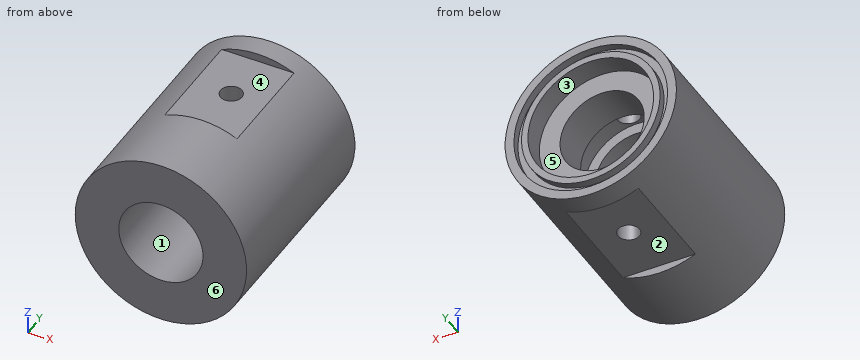
Autodesk Inventor part; units mm, degrees
ref_plane "YZ Plane" through (0, 0, 0) normal (1, 0, 0) x (0, 1, 0)
ref_plane "XZ Plane" through (0, 0, 0) normal (0, 1, 0) x (-1, 0, 0)
ref_plane "XY Plane" through (0, 0, 0) normal (0, 0, 1) x (1, 0, 0)
sketch "Sketch1" plane through (0, 0, 0) normal (0, 1, 0) x (-1, 0, 0)
  circle A0 centre (0, 0) radius 16
  dimension "d0" = 32
extrude "Extrusion1" add sketch "Sketch1" along normal blind 38
thread "Thread1"
sketch "Sketch2" plane through (0, 0, 0) normal (0, -1, 0) x (1, 0, 0)
  circle A0 centre (0, 0) radius 7.875
  dimension "d5" = 15.75
extrude "Extrusion2" cut sketch "Sketch2" against normal through all
sketch "Sketch3" plane through (0, 38, 0) normal (0, 1, 0) x (1, 0, 0)
  circle A0 centre (0, 0) radius 11.75
  dimension "d8" = 23.5
extrude "Extrusion3" cut sketch "Sketch3" against normal blind 4
sketch "Sketch4" plane through (0, 0, 0) normal (1, 0, 0) x (0, 1, 0)
  line L0 (0, 16) -> (38, 16)
  line L1 (34, 16) -> (14, 16)
  line L2 (14, 16) -> (14, 14.5)
  line L3 (14, 14.5) -> (34, 14.5)
  line L4 (34, 14.5) -> (34, 16)
  line L5 (0, -16) -> (38, -16)
  line L6 (34, -16) -> (14, -16)
  line L7 (14, -16) -> (14, -14.5)
  line L8 (14, -14.5) -> (34, -14.5)
  line L9 (34, -14.5) -> (34, -16)
  line L10 (38, -16) -> (38, 16)
  point P0 (0, 0)
  point P1 (14, 16)
  point P2 (14, -16)
  dimension "d11" = 20
  dimension "d12" = 1.5
  dimension "d13" = 1.5
  dimension "d33" = 4
extrude "Extrusion4" cut sketch "Sketch4" along normal through all both and the other way through all
sketch "Sketch5" plane through (0, 0, 0) normal (0, 0, 1) x (1, 0, 0)
  line L0 (7.875, 0) -> (7.875, 34)
  line L1 (7.875, 26.75) -> (9.875, 26.75)
  line L2 (9.875, 26.75) -> (9.875, 21.75)
  line L3 (9.875, 21.75) -> (7.875, 21.75)
  line L4 (7.875, 21.75) -> (7.875, 26.75)
  line L5 (0, -5.7834) -> (0, 45.928)
  line L6 (-11.75, 38) -> (11.75, 38)
  point P0 (0, 0)
  point P1 (7.875, 21.75)
  dimension "d17" = 11.25
  dimension "d18" = 16.25
  dimension "d19" = 2
revolve "Revolution1" cut sketch "Sketch5" angle 360 about axis through (0, -5.7834, 0) along (0, 1, 0)
sketch "Sketch6" plane through (6.7639, 34, -14.5) normal (0, 0, -1) x (-1, 0, 0)
  line L0 (-3.1111, -7.25) -> (16.6389, -7.25)
  line L1 (-3.1111, -12.25) -> (16.6389, -12.25)
  point P0 (6.7639, -34)
  point P1 (6.5383, -9.75)
  dimension "d20" = 5
  dimension "d21" = 2.5
hole "Hole1" at (0.2255, 24.25, -14.5) direction (0, 0, 1) diameter 4 end through all
sketch "Sketch7" plane through (0, 38, 0) normal (0, 1, 0) x (1, 0, 0)
  circle A0 centre (0, 0) radius 12.95
  circle A1 centre (0, 0) radius 14.35
  circle A2 centre (0, 0) radius 11.75
  dimension "d29" = 1.2
  dimension "d30" = 1.4
extrude "Extrusion5" cut sketch "Sketch7" against normal blind 1.4 contours A1
properties part number "Passthrough Base Insert" material "Aluminum 6061"
Can you work these out from the model? Positions are in its coordinate system, mm. Face numbers are marked on the shaded views. A direction names the side the tool comes from. Coordinates: 2 decimals unless noted, no trailing zeros. Loops run counter-clockwise (first coordinate to the right, second up) from the corner with the lowest first, then second, coordinate; pieces in that order, holes last. Notation, with made-up numbers: (85.5, 67) - (93.5, 67) arc R17 ccw to (93.5, 97) - close; hole circle Ø6 at (64, 11.25). An arc over 180 degrees is marked (long way). Answer as CSV lines item,"result". Start each with the question number.
1) Suppose I cut it at D-D (x = -1). Count the separate pieces of the cut face and the enclosed holes in it, plus the area to 3 significant figures.
2) Thinking about a two-plate mould opening in Z: for the marked faces 1, 2, 3 and 4, which applies, pulls with the +Z half, pulls with the -Z half, needs draft (parallel to the pull), parting line crosses it, or undercut?
3) Suppose I cut it at A-A (z = 0). Please give me the cut outline in (x, y) (3 decimals).
4) I need wall thicknesses on line 1 (Z direction, x = -0.5, y = 36.5); line 2 (Z direction, x = 0, y = 28) (3 decimals); line 3 (Y direction, x = -5.5, z = 6.5). Which ranges of each line are inside material? Lowest first, please. Write a range as from..to.
5) For pin 1 (0.5 mm diameter, centred on x = -2, z = 15, fed in from -Y); pin 2 (3 mm diameter, centred on x = 8.5, y = 15, fed in from -Z); pin 3 (5 mm diameter, centred on x = -13, y = 17.5, fed in from +Z); pin 4 (1.5 mm diameter, centred on y = 5, z = -4, fed in from -X), each with a flat end and sliding along its axis, tell me the tip position at first contact or that it passes through.
6) Suppose I cut it at C-C (y = 23.5). Please give me the cut outline in (x, z) (3 decimals), plus the area to 3 significant figures.
7) Which directions (+Z, -Z, +X, -X, +Y, -Y) give clear straight access to the entire face, cutting with the end or side of a thin tool? Please do the marked faces 5 and 6.
8) Suppose I cut it at B-B (y = 19). Please give me the cut outline in (x, z) (3 decimals), plus the area to 3 significant figures.
Check result:
1,separate pieces,"4"
1,enclosed holes,"0"
1,area,"476 mm²"
2,face 1,"undercut"
2,face 2,"pulls with the -Z half"
2,face 3,"undercut"
2,face 4,"pulls with the +Z half"
3,outline,"(-16, 0) - (-7.875, 0) - (-7.875, 21.75) - (-9.875, 21.75) - (-9.875, 26.75) - (-7.875, 26.75) - (-7.875, 34) - (-11.75, 34) - (-11.75, 38) - (-12.95, 38) - (-12.95, 36.6) - (-14.35, 36.6) - (-14.35, 38) - (-16, 38) - close; (7.875, 0) - (16, 0) - (16, 38) - (14.35, 38) - (14.35, 36.6) - (12.95, 36.6) - (12.95, 38) - (11.75, 38) - (11.75, 34) - (7.875, 34) - (7.875, 26.75) - (9.875, 26.75) - (9.875, 21.75) - (7.875, 21.75) - close"
4,line 1,"z = -15.99..-11.74, 11.74..15.99"
4,line 2,"z = -14.5..-7.875, 7.875..14.5"
4,line 3,"y = 0..21.75, 26.75..34"
5,pin 1,"stops at y = 0"
5,pin 2,"stops at z = -14.39"
5,pin 3,"stops at z = 12.07"
5,pin 4,"stops at x = -15.67"
6,outline,"(-6.764, -14.5) - (-1.629, -14.5) - (-1.629, -9.74) arc R9.875 cw to (-1.629, 9.74) - (-1.629, 14.5) - (-6.764, 14.5) arc R16 ccw to start; (2.08, -14.5) - (6.764, -14.5) arc R16 ccw to (6.764, 14.5) - (2.08, 14.5) - (2.08, 9.654) arc R9.875 cw to (2.08, -9.654) - close"
6,area,"436 mm²"
7,face 5,"+Y"
7,face 6,"+Z, -Z, +X, -X, -Y"
8,outline,"(-6.764, -14.5) - (6.764, -14.5) arc R16 ccw to (6.764, 14.5) - (-6.764, 14.5) arc R16 ccw to start; hole circle Ø15.75 at (0, 0)"
8,area,"582 mm²"
